Answer from the drawing. Dimensions are ordinates in mm from the lowest x, y and z of the part. A direction names the side the tool comes from. Coordinates: 2 decimals unless noted, no trailing zeros. Order: outer loops, then holes, each group sorted by start corner. A loop starts at its lowest first (then second) coordinate and runs counter-clockwise, first axis right, second up. Notation, with made-up numbers: (-38, -16.5) - (18, -16.5) arc R14 ccw to (18, 0.5) - close; hole circle Ø4 at (33.5, 48). An arc over 180 degrees is marked (long way). Answer as a JSON object with one key per item and string values. Group by question number.
1) A tool of negligible diameter and unlimited length cuts with its end or side. For the marked faces 5 and 6, from which of +Z, -Z, +X, -X, +Y, -Y can it reach the whole face along a straight path? Write none if from no direction.
2) This flat-tipped pin is pushed along its axis until it touches: P1, Ø1, axis at x = 67.5, z = 4.5, coming from the +Y side. Where does it stop, or does it pass through?
3) Section B-B (y = 12.7) is taken. Give the vertices of the cut face in (x, z).
4) Section C-C (z = 2.5) is taken. Count the separate pieces of the cut face and the enclosed holes in it, plus the area to 3 significant figures.
5) The mould has two halves that part along X. Classify the marked faces 1, 2, 3 and 4: released by +X, released by -X, zero draft, split by the parting line, or undercut.
6) Find the intervals of material crossed by line 1 along Y through (x, z) = (6.35, 4.75) (1 decimal); line 2 along X through (y, z) = (35.5, 0.5), in increasing order.
7) Section D-D (x = 56) is taken. Give the vertices of the cut face in (y, z), plus the area to 3 significant figures.
8) Section A-A (y = 26.5) is taken. Give the vertices of the cut face in (x, z).
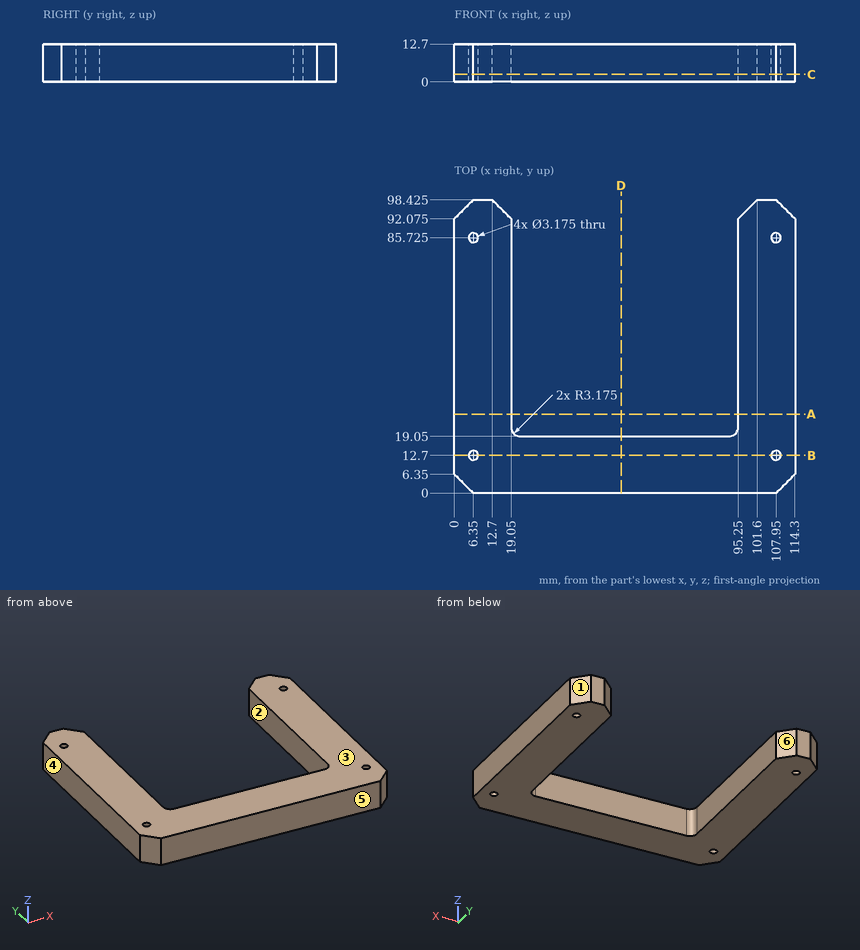
Report:
{
 "1": {"face 5": "+Z, -Z, +X, -X, -Y", "face 6": "+Z, -Z, +Y"},
 "2": {"P1": "stops at y = 19.05"},
 "3": {"outline": "(0, 0) - (4.76, 0) - (4.76, 12.7) - (0, 12.7) - close; (7.94, 0) - (106.36, 0) - (106.36, 12.7) - (7.94, 12.7) - close; (109.54, 0) - (114.3, 0) - (114.3, 12.7) - (109.54, 12.7) - close"},
 "4": {"separate pieces": "1", "enclosed holes": "4", "area": "5,050 mm²"},
 "5": {"face 1": "released by +X", "face 2": "undercut", "face 3": "zero draft", "face 4": "released by -X"},
 "6": {"line 1": "y = 0 to 11.1, 14.3 to 84.1, 87.3 to 98.4", "line 2": "x = 0 to 19.05, 95.25 to 114.3"},
 "7": {"outline": "(0, 0) - (19.05, 0) - (19.05, 12.7) - (0, 12.7) - close", "area": "242 mm²"},
 "8": {"outline": "(0, 0) - (19.05, 0) - (19.05, 12.7) - (0, 12.7) - close; (95.25, 0) - (114.3, 0) - (114.3, 12.7) - (95.25, 12.7) - close"}
}
